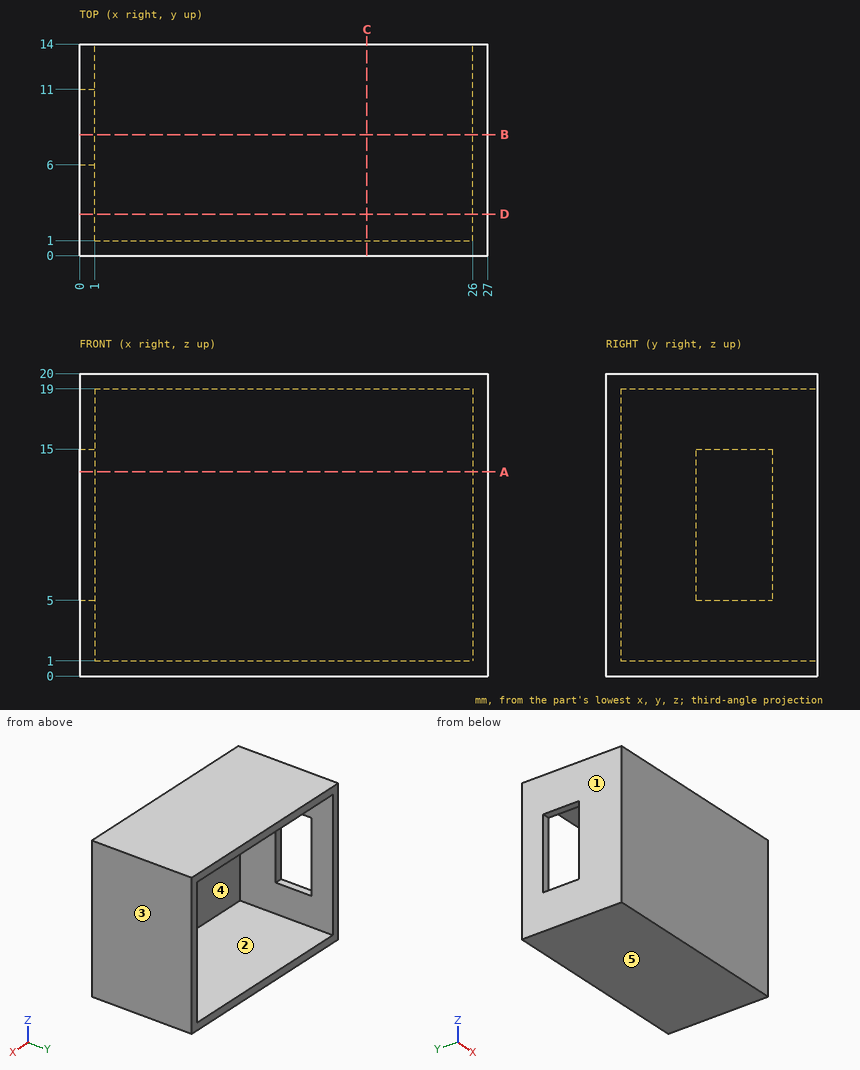
For this review, use the dimensioned drawing (mm, ordinates from the lowest corner) and the shaded views. A direction names the side the tool comes from. Coordinates: 2 decimals unless noted, no trailing zeros. Write each loop counter-clockwise with the first axis right and the second up, starting at its lowest first coordinate (ties: lowest second). Pieces come first, ordered by that corner, then holes. Notation, with made-up numbers: (-16, 39) -> (40, 39) arc R11 cw to (40, 43) -> close; hole circle Ø10 at (43.5, 34). An arc over 180 degrees is marked (long way). Write each question's results on one line, items separated by ' | '. Start each with the question number.
(1) Take a section at D-D on y = 2.75. Write out the cut boundary in (x, z), and give its area (3 significant figures).
(2) Take a section at B-B on y = 8. Write out the cut boundary in (x, z), and give its area (3 significant figures).
(3) The part is to be moulded in two halves that separate along X. For the marked faces 3, 4 and 5, say which applies: pulls with the +X half, pulls with the -X half, needs draft (parallel to the pull), parting line crosses it, or undercut.
(4) Clearance check with a flat-ended pin moving along its axis: P1, Ø1, axis at x = 11.5, z = 3, coming from the +Y side. State where the tip first meets the part, or that it passes through.
(5) For line 1 along X through (y, z) = (12, 18.25); line 2 along Z through (x, y) = (25, 11.5); line 3 along Y through (x, z) = (2.25, 18.75), list the stretches that pass through material, from the lowest coordinate up. Write a range as from..to.
(6) Tool access review of the marked faces 1 and 2: name each direction out of +Z, -Z, +X, -X, +Y, -Y from which nothing blocks a thin tool from reaching the whole face with its end or side.
(7) Take a section at A-A on z = 13.5. Write out the cut boundary in (x, y), and give its area (3 significant figures).
(8) Take a section at C-C on x = 19. Write out the cut boundary in (y, z).
Results found:
1) outline: (0, 0) -> (27, 0) -> (27, 20) -> (0, 20) -> close; hole (1, 1) -> (26, 1) -> (26, 19) -> (1, 19) -> close | area: 90.0 mm2
2) outline: (0, 0) -> (27, 0) -> (27, 20) -> (0, 20) -> (0, 15) -> (1, 15) -> (1, 19) -> (26, 19) -> (26, 1) -> (1, 1) -> (1, 5) -> (0, 5) -> close | area: 80.0 mm2
3) face 3: pulls with the +X half | face 4: undercut | face 5: needs draft
4) P1: stops at y = 1
5) line 1: x = 0..1, 26..27 | line 2: z = 0..1, 19..20 | line 3: y = 0..1
6) face 1: +Z, -Z, -X, +Y, -Y | face 2: +Y
7) outline: (0, 0) -> (27, 0) -> (27, 14) -> (26, 14) -> (26, 1) -> (1, 1) -> (1, 6) -> (0, 6) -> close; (0, 11) -> (1, 11) -> (1, 14) -> (0, 14) -> close | area: 48.0 mm2
8) outline: (0, 0) -> (14, 0) -> (14, 1) -> (1, 1) -> (1, 19) -> (14, 19) -> (14, 20) -> (0, 20) -> close
